```python
from build123d import *

# Parameters (mm, degrees)
PAD_DEPTH    = 10
SKETCH001_R  = 13
PAD001_DEPTH = 20
POCKET_DEPTH = 15


with BuildPart() as part:
    # Sketch → Pad (new body)
    with BuildSketch(Plane.XY):
        Polygon((0, 9.298454), (-9.298454, 0), (0, -9.298454), (9.298454, 0), align=None)
    extrude(amount=PAD_DEPTH)

    # Sketch001 (on Face6 of Pad) → Pad001 (join)
    with BuildSketch(Plane.XY.offset(10)):
        Circle(SKETCH001_R)
    extrude(amount=PAD001_DEPTH)

    # Sketch002 (on Face3 of Pad001) → Pocket (cut)
    with BuildSketch(Plane.XY.offset(30)):
        Polygon((0, 9.64), (-8.348485, 4.82), (-8.348485, -4.82), (0, -9.64), (8.348485, -4.82), (8.348485, 4.82), align=None)
    extrude(amount=-POCKET_DEPTH, mode=Mode.SUBTRACT)


solid = part.part
```
Build history of the part. All positions in model axes, mm. A direction names the side the tool comes from. Coordinates: 2 decimals unless noted, no trailing zeros. Order: outer loops, then holes, each group sorted by start corner. A loop starts at its lowest first (then second) coordinate and runs counter-clockwise, first axis right, second up. Notation, with made-up numbers: (31, 30.5) -> (37, 30.5) arc R17 ccw to (37, 46.5) -> close; hole circle Ø11 at (-37, 80). An arc over 180 degrees is marked (long way). Answer in a Markdown table with one row per item. Add a question column.
Q1. Band-saw the part on C-C, the plane x = -5.5. List the corners of the cut face in (y, z), then the cut area to 3 significant figures.
Q2. Band-saw the part on D-D, the plane z = 12.25. List the corners of the cut face in (x, y), then the cut area to 3 significant figures.
Q3. Which spindle directions (+Z, -Z, +X, -X, +Y, -Y) get a long thin tool onto all of the face, cutting with end or side? Do faces 4 (the face through (4.6, -4.7, 4.9)), 5 (the face through (-4.6, 4.7, 4.9)), 6 (the face through (-4.12, 7.26, 22.6)). Say none if no direction does.
Q4. Band-saw the part on A-A, the plane z = 23. List the corners of the cut face in (x, y).
Q5. Drop flat-ended pins along their axis: pin 1 (1.5 mm diameter, centred on y = 9.5, z = 5.5, fed in from -X); pin 2 (5 mm diameter, centred on y = -7, z = 5.5, fed in from +X); pin 3 (2 mm diameter, centred on y = -1.5, z = 9.5, fed in from +X). Give the stop position or say it passes through.
Q6. Band-saw the part on B-B, the plane y = -3.25. List the corners of the cut face in (x, z).
Q7. Mould opens along Y. For faces 1 (the face through (0, 0, 0)), 2 (the face through (4.7, 4.6, 4.9)), 3 (the face through (0, 0, 15)) say: +Y half, -Y half, draft (parallel to the pull), parting line (faces both ways), or undercut.
Q8. Wall check: line 1 along Z through (x, y) = (-10.75, 4.25); line 2 along Z through (x, y) = (-5.5, 2); line 3 along X through (y, z) = (-0.25, 17.75). Give the ranges that are in metal, low to high. Write a range as [from, to].
Answers follow:
| question | item | result |
|---|---|---|
| 1 | outline | (-11.78, 10) -> (-3.8, 10) -> (-3.8, 0) -> (3.8, 0) -> (3.8, 10) -> (11.78, 10) -> (11.78, 30) -> (6.46, 30) -> (6.46, 15) -> (-6.46, 15) -> (-6.46, 30) -> (-11.78, 30) -> close |
| 1 | area | 353 mm^2 |
| 2 | outline | circle Ø26 at (0, 0) |
| 2 | area | 531 mm^2 |
| 3 | face 4 | -Z, +X, -Y |
| 3 | face 5 | -Z, -X, +Y |
| 3 | face 6 | +Z |
| 4 | outline | circle Ø26 at (0, 0); hole (-8.35, -4.82) -> (0, -9.64) -> (8.35, -4.82) -> (8.35, 4.82) -> (0, 9.64) -> (-8.35, 4.82) -> close |
| 5 | pin 1 | x = -0.55 |
| 5 | pin 2 | x = 4.8 |
| 5 | pin 3 | x = 12.98 |
| 6 | outline | (-12.59, 10) -> (-6.05, 10) -> (-6.05, 0) -> (6.05, 0) -> (6.05, 10) -> (12.59, 10) -> (12.59, 30) -> (8.35, 30) -> (8.35, 15) -> (-8.35, 15) -> (-8.35, 30) -> (-12.59, 30) -> close |
| 7 | face 1 | draft |
| 7 | face 2 | +Y half |
| 7 | face 3 | undercut |
| 8 | line 1 | [10, 30] |
| 8 | line 2 | [0, 15] |
| 8 | line 3 | [-13, -8.35], [8.35, 13] |
